Input: part model. Units: mm. Frame: model coordinates. Coordinates: 2 decimals unless noted, no trailing zeros. Loops run counter-clockwise (first coordinate to the right, second up) from the corner with the lowest first, then second, coordinate; pieces in that order, holes last.
Item 1: Section A-A on z = 6.35. Return loops of the section in (x, y) (3 decimals), and give its area (3 significant figures).
Item 2: Contact query for flat-ended pins moving along their axis: P1, Ø3, axis at x = 48, y = -7.5, coming from the -Z side; P2, Ø1, axis at y = -8, z = -5, coming from the -X side. Output: stop coordinate, or through.
Item 3: Section B-B on y = -3.75. Return loops of the section in (x, z) (3 decimals).
Item 4: Ray query, line 1 along Z through (x, y) = (40, -9); line 2 along Z through (x, y) = (203.5, -1.5); line 3 along Z through (x, y) = (42.5, -2.75). Return the intervals inside material, ascending.
Item 5: Section D-D on x = 73. Return loops of the section in (y, z), and give its area (3 significant figures).
Item 6: Section C-C on x = 203.2. Return loops of the section in (y, z) (3 decimals), and give its area (3 significant figures).
```python
from build123d import *

# Parameters (mm, degrees)
F0_R     = 9.525
F1_DEPTH = 10
F2_SIZE  = 1.016


# Not quite as in the source:
# - a feature names something its author has since deleted; it is built from what else it names


with BuildPart() as f1:
    # F0 (on Front) → F1 (new body)
    with BuildSketch(Plane.XZ):
        Polygon((0, 38.1), (0, 0), (76.2, 0), (76.2, -9.525), (120.65, -19.05), (228.6, -19.05), (228.6, 31.75), (104.775, 69.85), (31.75, 69.85), align=None)
        with Locations((203.2, 6.35)):
            Circle(F0_R, mode=Mode.SUBTRACT)
    extrude(amount=F1_DEPTH)

    # F2
    f2_edges = [f1.edges().sort_by_distance(p)[0] for p in [
        (15.875, -10, 53.975),
        (0, -10, 19.05),
        (38.1, -10, 0),
        (76.2, -10, -4.7625),
        (98.425, -10, -14.2875),
        (174.625, -10, -19.05),
        (228.6, -10, 6.35),
        (166.6875, -10, 50.8),
        (68.2625, -10, 69.85),
        (193.675, -10, 6.35),
        (15.875, 0, 53.975),
        (0, 0, 19.05),
        (38.1, 0, 0),
        (76.2, 0, -4.7625),
        (98.425, 0, -14.2875),
        (174.625, 0, -19.05),
        (228.6, 0, 6.35),
        (166.6875, 0, 50.8),
        (68.2625, 0, 69.85),
        (193.675, 0, 6.35),
    ]]
    chamfer(f2_edges, length=F2_SIZE)


solid = f1.part
```
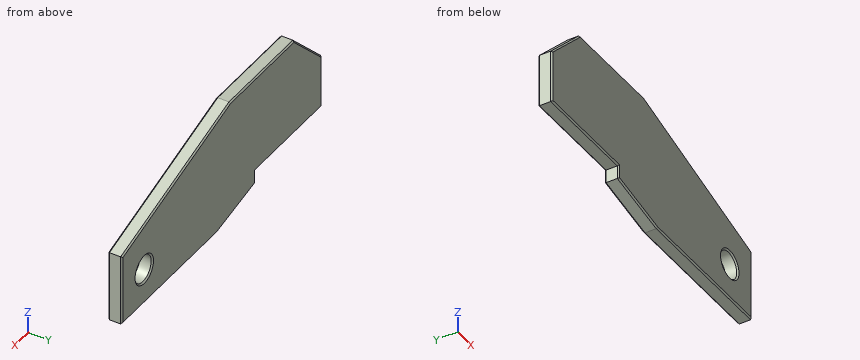
Results found:
1. outline: (0, -8.984) - (1.016, -10) - (192.659, -10) - (193.675, -8.984) - (193.675, -1.016) - (192.659, 0) - (1.016, 0) - (0, -1.016) - close; (212.725, -8.984) - (213.741, -10) - (227.584, -10) - (228.6, -8.984) - (228.6, -1.016) - (227.584, 0) - (213.741, 0) - (212.725, -1.016) - close
1. area: 2,090 mm2
2. P1: stops at z = 0
2. P2: stops at x = 76.2
3. outline: (0, 0) - (76.2, 0) - (76.2, -9.525) - (120.65, -19.05) - (228.6, -19.05) - (228.6, 31.75) - (104.775, 69.85) - (31.75, 69.85) - (0, 38.1) - close; hole circle Ø19.05 at (203.2, 6.35)
4. line 1: z = 0.02 to 69.83
4. line 2: z = -19.05 to -3.17, 15.87 to 39.47
4. line 3: z = 0 to 69.85
5. outline: (-10, 1.02) - (-8.98, 0) - (-1.02, 0) - (0, 1.02) - (0, 68.83) - (-1.02, 69.85) - (-8.98, 69.85) - (-10, 68.83) - close
5. area: 696 mm2
6. outline: (-10, -18.034) - (-8.984, -19.05) - (-1.016, -19.05) - (0, -18.034) - (0, -4.191) - (-1.016, -3.175) - (-8.984, -3.175) - (-10, -4.191) - close; (-10, 16.891) - (-8.984, 15.875) - (-1.016, 15.875) - (0, 16.891) - (0, 38.502) - (-1.016, 39.565) - (-8.984, 39.565) - (-10, 38.502) - close
6. area: 391 mm2
